from build123d import *

# Parameters (mm, degrees)
F1_DEPTH  = 25.4
F2_R      = 3.175
F4_DEPTH  = 32.259
F5_R      = 6.35
F6_W      = 61.087
F6_H      = 12.7
F7_DEPTH  = 3.175
F8_R      = 3.175
F9_W      = 22.86
F9_H      = 3.175
F10_DEPTH = 25.4
F11_R     = 1.524


with BuildPart() as f1:
    # F0 (on Top) → F1 (new body)
    with BuildSketch(Plane.XY):
        Polygon((-30.5435, 29.083), (0, 29.083), (30.5435, 29.083), (30.5435, 0), (59.1185, 0), (59.1185, 3.175), (33.7185, 3.175), (33.7185, 32.258), (0, 32.258), (-33.7185, 32.258), (-33.7185, 3.175), (-59.1185, 3.175), (-59.1185, 0), (-30.5435, 0), align=None)
    extrude(amount=F1_DEPTH)

    # F2
    f2_edges = [f1.edges().sort_by_distance(p)[0] for p in [
        (-30.5435, 0, 12.7),
        (30.5435, 0, 12.7),
    ]]
    fillet(f2_edges, radius=F2_R)

    # F3 (on Front) → F4 (cut, through all)
    with BuildSketch(Plane.XZ):
        with BuildLine():
            ThreePointArc((-48.8315, 7.8105), (-46.4185, 5.3975), (-44.0055, 7.8105))
            Line((-44.0055, 7.8105), (-44.0055, 17.4625))
            ThreePointArc((-44.0055, 17.4625), (-46.4185, 19.8755), (-48.8315, 17.4625))
            Line((-48.8315, 17.4625), (-48.8315, 7.8105))
        make_face()
        with BuildLine():
            ThreePointArc((48.8315, 17.4498), (46.4185, 19.8628), (44.0055, 17.4498))
            Line((44.0055, 17.4498), (44.0055, 7.7978))
            ThreePointArc((44.0055, 7.7978), (46.4185, 5.3848), (48.8315, 7.7978))
            Line((48.8315, 7.7978), (48.8315, 17.4498))
        make_face()
    extrude(amount=-F4_DEPTH, mode=Mode.SUBTRACT)

    # F5
    f5_edges = [f1.edges().sort_by_distance(p)[0] for p in [
        (-59.1185, 1.5875, 0),
        (-59.1185, 1.5875, 25.4),
        (59.1185, 1.5875, 25.4),
        (59.1185, 1.5875, 0),
    ]]
    fillet(f5_edges, radius=F5_R)

    # F6 (on face) → F7 (join)
    with BuildSketch(Plane(origin=(0, 0, 0), x_dir=(1, 0, 0), z_dir=(0, 0, -1))):
        with Locations((0, -22.733)):
            Rectangle(F6_W, F6_H)
    extrude(amount=-F7_DEPTH)

    # F8
    f8_edges = [f1.edges().sort_by_distance(p)[0] for p in [
        (33.7185, 3.175, 12.7),
        (33.7185, 32.258, 12.7),
        (-33.7185, 32.258, 12.7),
        (-33.7185, 3.175, 12.7),
        (30.5435, 16.383, 1.5875),
        (-30.5435, 16.383, 1.5875),
    ]]
    fillet(f8_edges, radius=F8_R)

    # F9 (on face) → F10 (cut)
    with BuildSketch(Plane.XY.offset(3.175)):
        with Locations((0, 17.9705)):
            Rectangle(F9_W, F9_H)
    extrude(amount=-F10_DEPTH, mode=Mode.SUBTRACT)

    # F11
    f11_edges = [f1.edges().sort_by_distance(p)[0] for p in [
        (-11.43, 16.383, 1.5875),
        (11.43, 16.383, 1.5875),
    ]]
    fillet(f11_edges, radius=F11_R)


solid = f1.part
Geometry check sheet. Reference: the model listing, model coordinates, mm. A direction names the side the tool comes from. Coordinates: 2 decimals unless noted, no trailing zeros. Order: outer loops, then holes, each group sorted by start corner. A loop starts at its lowest first (then second) coordinate and runs counter-clockwise, first axis right, second up. Notation, with made-up numbers: (-22.75, 38.25) - (20.25, 38.25) arc R35 cw to (20.25, 75.25) - close; hole circle Ø7 at (40.25, 72). An arc over 180 degrees is marked (long way). One line per item, written item: value.
(1) Depth check by flat-ended pin: pin 1 Ø12 at (x, y) = (-23.5, 7.5) entering from +Z; pin 2 Ø12.5 at (x, y) = (-13.5, 22) entering from +Z (3 decimals); pin 3 Ø11.5 at (y, z) = (15.5, 10) entering from -X; pin 4 Ø12 at (x, z) = (5, 17) entering from -Y. Enter the tip coordinate at first touch or a pass-through.
Data:
pin 1: passes through
pin 2: stops at z = 3.175
pin 3: stops at x = -33.72
pin 4: stops at y = 29.08
(2) Thickness scan on probe 1 along X at (y, z) = (27.5, 11.75); probe 2 along Z at (x, y) = (6, 20) (3 decimals); probe 3 along Y at (x, z) = (1.5, 17.25). Record the ranges inside material, lowest first. Write a range as from..to.
Data:
probe 1: x = -33.72..-30.54, 30.54..33.72
probe 2: z = 0..3.175
probe 3: y = 29.08..32.26
(3) Release check for a two-part mould opening along Z. For faces 5 (the face through (-57.2, 1.6, 23.6)), 6 (the face through (44.006, 2, 13)), 7 (the face through (-46.365, 1.565, 19.875)), 8 (the face through (30.544, 16, 13)) record: +Z half, -Z half, draft (parallel to the pull), parting line (faces both ways), or undercut.
Data:
face 5: +Z half
face 6: undercut
face 7: undercut
face 8: draft
(4) Access from +Z, -Z, +X, -X, +Y, -Y to the whole of each face (thin tool, end or side, straight path). Record for faces 1 (the face through (-46.5, 1.6, 5.4)), 2 (the face through (51, 3.175, 13)), 3 (the face through (-20, 16.383, 2)), 4 (the face through (-30.544, 16, 13)).
Data:
face 1: +Y, -Y
face 2: +Z, -Z, +X, +Y
face 3: +Z, -Z, -Y
face 4: +Z, -Y
(5) Sectioned sample at C-C (y = 28). Enter the section's corners in (x, z) (1 decimal), and give its area (3 significant figures).
Data:
outline: (-33.7, 0) - (33.7, 0) - (33.7, 25.4) - (30.5, 25.4) - (30.5, 3.2) - (-30.5, 3.2) - (-30.5, 25.4) - (-33.7, 25.4) - close
area: 355 mm^2
(6) Sectioned sample at D-D (x = 46). Enter the section's corners in (y, z) (3 decimals).
Data:
outline: (0, 0) - (3.175, 0) - (3.175, 5.421) - (0, 5.421) - close; (0, 19.826) - (3.175, 19.826) - (3.175, 25.4) - (0, 25.4) - close
(7) Sectioned sample at B-B (y = 11). Enter the section's corners in (x, z), and give its area (3 significant figures).
Data:
outline: (-33.72, 0) - (-30.54, 0) - (-30.54, 25.4) - (-33.72, 25.4) - close; (30.54, 0) - (33.72, 0) - (33.72, 25.4) - (30.54, 25.4) - close
area: 161 mm^2
(8) Sectioned sample at A-A (z = 11). Count the separate pieces of the cut face and the enclosed holes in it, and give its area (3 significant figures).
Data:
separate pieces: 3
enclosed holes: 0
area: 525 mm^2
